from build123d import *

# Parameters (mm, degrees)
SKETCH1_W           = 6.35
SKETCH1_H           = 6.35
SKETCH1_R           = 3.6703
BOSS_EXTRUDE1_DEPTH = 6.35


with BuildPart() as part:
    # Sketch1 → Boss-Extrude1 (new body)
    with BuildSketch(Plane(origin=(0, 0, 0), x_dir=(1, 0, 0), z_dir=(0, 1, 0))):
        Polygon((0, 25.4), (0, 0), (20.0406, 0), (20.0406, 25.4), (13.6906, 25.4), (13.6906, 44.45), (20.0406, 44.45), (20.0406, 69.85), (0, 69.85), (0, 44.45), (6.35, 44.45), (6.35, 25.4), align=None)
        with Locations((10.0203, 6.35)):
            Rectangle(SKETCH1_W, SKETCH1_H, mode=Mode.SUBTRACT)
        with Locations((10.0203, 22.225)):
            Circle(SKETCH1_R, mode=Mode.SUBTRACT)
        with Locations((10.0203, 63.5)):
            Rectangle(SKETCH1_W, SKETCH1_H, mode=Mode.SUBTRACT)
        with Locations((10.0203, 47.625)):
            Circle(SKETCH1_R, mode=Mode.SUBTRACT)
    extrude(amount=BOSS_EXTRUDE1_DEPTH)


solid = part.part
Model file for the job. Use its own axes, mm. A direction names the side the tool comes from. Give positions to 0.01 mm unless a question says otherwise; leave off trailing zeros. Loops run counter-clockwise (first coordinate to the right, second up) from the corner with the lowest first, then second, coordinate; pieces in that order, holes last.
Item 1: Drill centre lines: line 1 along X through (y, z) = (3.25, -6); line 2 along Z through (x, y) = (2.25, 4.25); line 3 along Z through (x, y) = (13.25, 5.5). Where is each one in solid material? Low to high.
Check values:
line 1: x = 0 to 6.85, 13.2 to 20.04
line 2: z = -69.85 to -44.45, -25.4 to 0
line 3: z = -69.85 to -49.37, -45.88 to -23.97, -20.48 to 0
Item 2: Which spindle directions (+Z, -Z, +X, -X, +Y, -Y) get a long thin tool onto all of the face, cutting with end or side? Do faces 4 (the face through (3, 3, -44.45)), 5 (the face through (17, 3, -44.45)), 6 (the face through (13.195, 3, -6)). Say none if no direction does.
Check values:
face 4: -X, +Y, -Y
face 5: +X, +Y, -Y
face 6: +Y, -Y
Item 3: Slice it at A-A (x = 18.5). Write the cut outline in (y, z).
Check values:
outline: (0, -69.85) - (6.35, -69.85) - (6.35, -44.45) - (0, -44.45) - close; (0, -25.4) - (6.35, -25.4) - (6.35, 0) - (0, 0) - close
Item 4: Mould opens along X. For faces 1 (the face through (13.691, 3, -35)), 2 (the face through (10, 3, -66.675)), 3 (the face through (10, 0, -35)) say: +X half, -X half, draft (parallel to the pull), parting line (faces both ways), or undercut.
Check values:
face 1: +X half
face 2: undercut
face 3: draft
Item 5: Drop flat-ended pins along their axis: P1, Ø3, axis at y = 3.5, z = -38, coming from the +X side; P2, Ø11.5, axis at x = 10.02, z = -22.22, coming from the -Y side; P3, Ø3, axis at y = 0.5, z = -39, coming from the -X side. Give the stop position or say it passes through.
Check values:
P1: stops at x = 13.69
P2: stops at y = 0
P3: stops at x = 6.35
Item 6: Slice it at C-C (x = 12). Write the cut outline in (y, z) (3 decimals).
Check values:
outline: (0, -69.85) - (6.35, -69.85) - (6.35, -66.675) - (0, -66.675) - close; (0, -60.325) - (6.35, -60.325) - (6.35, -50.716) - (0, -50.716) - close; (0, -44.534) - (6.35, -44.534) - (6.35, -25.316) - (0, -25.316) - close; (0, -19.134) - (6.35, -19.134) - (6.35, -9.525) - (0, -9.525) - close; (0, -3.175) - (6.35, -3.175) - (6.35, 0) - (0, 0) - close
Item 7: Slice it at B-B (y = 3.75). Write the cut outline in (x, z) (3 decimals), plus the area to 3 significant figures.
Check values:
outline: (0, -69.85) - (20.041, -69.85) - (20.041, -44.45) - (13.691, -44.45) - (13.691, -25.4) - (20.041, -25.4) - (20.041, 0) - (0, 0) - (0, -25.4) - (6.35, -25.4) - (6.35, -44.45) - (0, -44.45) - close; hole circle Ø7.341 at (10.02, -47.625); hole circle Ø7.341 at (10.02, -22.225); hole (6.845, -66.675) - (13.195, -66.675) - (13.195, -60.325) - (6.845, -60.325) - close; hole (6.845, -9.525) - (13.195, -9.525) - (13.195, -3.175) - (6.845, -3.175) - close
area: 993 mm2
Item 8: Slice it at D-D (z = -36). Write the cut outline in (x, y).
Check values:
outline: (6.35, 0) - (13.69, 0) - (13.69, 6.35) - (6.35, 6.35) - close
